Read the model definition and answer for the solid it produces. Units are mm, in the model's axes. Give positions to 0.01 mm unless a question says otherwise; leave off trailing zeros. Write each loop counter-clockwise with the first axis right and the second up, starting at its lowest first coordinate (ties: lowest second). Pieces come first, ordered by that corner, then holes.
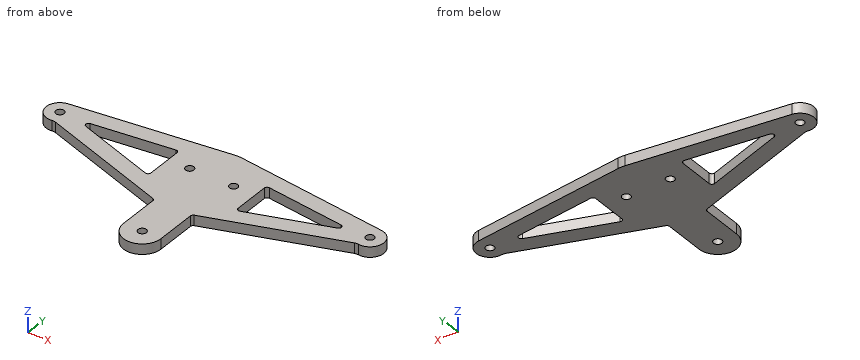
```python
from build123d import *

# Parameters (mm, degrees)
ESBO_O1_R                = 1.5
RESSALTO_EXTRUS_O1_DEPTH = 3.75
FILETE2_R                = 10


with BuildPart() as part:
    # Esboço1 → Ressalto-extrusão1 (new body)
    with BuildSketch(Plane.XY):
        with BuildLine():
            Line((56.5, 11.974876818), (-0.609346717, 4.962730758))
            ThreePointArc((-0.609346717, 4.962730758), (-4.956620044, -0.657204491), (0.705001075, -4.950047827))
            ThreePointArc((0.705001075, -4.950047827), (1.403511249, -4.932754227), (2.087076087, -5.077511421))
            Line((2.087076087, -5.077511421), (48.969691456, -20.895588778))
            ThreePointArc((48.969691456, -20.895588778), (49.462308887, -21.259883017), (49.65, -21.843110478))
            Line((49.65, -21.843110478), (49.65, -36.675123182))
            ThreePointArc((49.65, -36.675123182), (56.5, -43.525123182), (63.35, -36.675123182))
            Line((63.35, -36.675123182), (63.35, -21.843110478))
            ThreePointArc((63.35, -21.843110478), (63.537691113, -21.259883017), (64.030308544, -20.895588778))
            Line((64.030308544, -20.895588778), (110.912923913, -5.077511421))
            ThreePointArc((110.912923913, -5.077511421), (111.596488751, -4.932754227), (112.294998925, -4.950047827))
            ThreePointArc((112.294998925, -4.950047827), (117.956620044, -0.657204491), (113.609346717, 4.962730758))
            Line((113.609346717, 4.962730758), (56.5, 11.974876818))
        make_face()
        Circle(ESBO_O1_R, mode=Mode.SUBTRACT)
        with Locations((113, 0)):
            Circle(ESBO_O1_R, mode=Mode.SUBTRACT)
        with Locations((48.5, -1.675123182)):
            Circle(ESBO_O1_R, mode=Mode.SUBTRACT)
        with Locations((64.5, -1.675123182)):
            Circle(ESBO_O1_R, mode=Mode.SUBTRACT)
        with Locations((56.5, -36.675123182)):
            Circle(ESBO_O1_R, mode=Mode.SUBTRACT)
        with BuildLine():
            Line((39.280308544, -11.294106381), (10.609409181, -1.620616529))
            ThreePointArc((10.609409181, -1.620616529), (9.93425904, -0.571654218), (10.807231293, 0.319451323))
            Line((10.807231293, 0.319451323), (39.478130657, 3.839795112))
            ThreePointArc((39.478130657, 3.839795112), (40.262620048, 3.596204682), (40.6, 2.847248961))
            Line((40.6, 2.847248961), (40.6, -10.346584681))
            ThreePointArc((40.6, -10.346584681), (40.183227462, -11.158893568), (39.280308544, -11.294106381))
        make_face(mode=Mode.SUBTRACT)
        with BuildLine():
            Line((73.719691456, -11.294106381), (102.390590819, -1.620616529))
            ThreePointArc((102.390590819, -1.620616529), (103.06574096, -0.571654218), (102.192768707, 0.319451323))
            Line((102.192768707, 0.319451323), (73.521869343, 3.839795112))
            ThreePointArc((73.521869343, 3.839795112), (72.737379952, 3.596204682), (72.4, 2.847248961))
            Line((72.4, 2.847248961), (72.4, -10.346584681))
            ThreePointArc((72.4, -10.346584681), (72.816772538, -11.158893568), (73.719691456, -11.294106381))
        make_face(mode=Mode.SUBTRACT)
    extrude(amount=RESSALTO_EXTRUS_O1_DEPTH)

    # Filete2
    filete2_edges = [part.edges().sort_by_distance(p)[0] for p in [
        (56.5, 11.974876818, 1.875),
    ]]
    fillet(filete2_edges, radius=FILETE2_R)


solid = part.part
```
Item 1: Section C-C (y = -27.5) is taken. Write down the section's boundary in (x, z), and give its area (3 significant figures).
Result set:
outline: (49.65, 0) - (63.35, 0) - (63.35, 3.75) - (49.65, 3.75) - close
area: 51.4 mm2
Item 2: Find the intervals of material crossed by line 1 along Y through (x, z) = (48.5, 2.7); line 2 along Y through (x, z) = (113, 1.05); line 3 along X through (y, z) = (-29, 0.2), in increasing order.
Result set:
line 1: y = -20.74 to -3.18, -0.18 to 10.99
line 2: y = -5 to -1.5, 1.5 to 5.04
line 3: x = 49.65 to 63.35
Item 3: Section B-B (z = 1.2) is taken. Give the number of separate pieces and of enclosed holes in the cut face, and give its area (3 significant figures).
Result set:
separate pieces: 1
enclosed holes: 7
area: 2,320 mm2
Item 4: Section D-D (x = 33) is taken. Write down the section's boundary in (y, z), and give its area (3 significant figures).
Result set:
outline: (-15.51, 0) - (-9.18, 0) - (-9.18, 3.75) - (-15.51, 3.75) - close; (3.04, 0) - (9.09, 0) - (9.09, 3.75) - (3.04, 3.75) - close
area: 46.4 mm2
Item 5: Section A-A (x = 56.5) is taken. Write down the section's boundary in (y, z), and give its area (3 significant figures).
Result set:
outline: (-43.53, 0) - (-38.18, 0) - (-38.18, 3.75) - (-43.53, 3.75) - close; (-35.18, 0) - (11.9, 0) - (11.9, 3.75) - (-35.18, 3.75) - close
area: 197 mm2
Item 6: Each of these flat-tipped pins is pushed along its axis until it touches: pin 1 Ø1 at (x, z) = (24, 3) entering from +Y; pin 2 Ø4 at (x, y) = (64.5, -1.68) entering from +Z; pin 3 Ø1.5 at (x, z) = (48.5, 1.5) entering from +Y; pin 4 Ø1 at (y, z) = (4.5, 2) entering from +X. Where does it stop, or does it pass through?
Result set:
pin 1: stops at y = 8.05
pin 2: stops at z = 3.75
pin 3: stops at y = 11.08
pin 4: stops at x = 116
